Can you work these out from the model? Positions are in its coordinate system, mm. Give positions to 0.01 mm unless a question says otherwise; leave off trailing zeros. Write each loop counter-clockwise with the first axis right and the second up, starting at its lowest first coordinate (ties: lowest second). Pieces come first, ordered by that corner, then holes.
1. Suppose I cut it at D-D (y = 25.5). Please give me the cut outline in (x, z).
2. Suppose I cut it at B-B (z = 0). Please give me the cut outline in (x, y) (3 decimals), and give its area (3 significant figures).
3. Suppose I cut it at A-A (x = 0). Please give me the cut outline in (y, z), and give its area (3 significant figures).
4. Suppose I cut it at C-C (y = 4). Please give me the cut outline in (x, z).
5. I'm going to push flat-ended pins straight in: pin 1 (1 mm diameter, centred on x = 30.5, z = -13.5, fed in from -Y); pin 2 (1.5 mm diameter, centred on x = 13, z = 2, fed in from -Y); pin 3 (6 mm diameter, centred on y = 6.5, z = -28, fed in from +X). Where does each tip first touch, or does it pass through?
6. If I drill on probe 1 along Z at (x, y) = (-28.5, 18); probe 2 along Z at (x, y) = (24, 21.5); probe 3 along X at (y, z) = (14, -20), over which ranges is the centre line in solid material (lowest first)?
```python
from build123d import *

# Parameters (mm, degrees)
SKETCH_2_R          = 9
SKETCH_2_R_2        = 5.000000000000001
SKETCH_2_R_3        = 7.999999999999998
SKETCH_2_R_4        = 6.124999999999995
CUT_EXTRUDE_1_DEPTH = 107.33743200790742


with BuildPart() as part:
    # Эскиз1 → Повернуть1 (revolve)
    with BuildSketch(Plane.XY, mode=Mode.PRIVATE) as revolve_1_sk:
        with BuildLine():
            Line((0, 39.36501550915903), (0, 36.36501550915897))
            ThreePointArc((0, 36.36501550915897), (32.17757492953397, 30.613071103520923), (60.369714413268355, 14.069659601627245))
            ThreePointArc((60.369714413268355, 14.069659601627245), (65.15206854111862, 7.74515045998565), (66.84999999999997, 1.388e-14))
            Line((66.84999999999997, 1.388e-14), (69.85000000000002, 1.388e-14))
            ThreePointArc((69.85000000000002, 1.388e-14), (67.87693354038171, 9.000184617206603), (62.31964058940756, 16.349525366887885))
            ThreePointArc((62.31964058940756, 16.349525366887885), (33.216902285139106, 33.427284785509414), (0, 39.36501550915903))
        make_face()
    revolve(revolve_1_sk.sketch.rotate(Axis((0, 69.55204547466519, 0), (0, -1, 0)), 90), axis=Axis((0, 69.55204547466519, 0), (0, -1, 0)))

    # Эскиз2 → Вырез-Вытянуть1 (cut, through all)
    with BuildSketch(Plane(origin=(0, 39.36501550915903, 0), x_dir=(1, 0, 0), z_dir=(0, 1, 0))):
        with Locations(Location((0, 0, 0), (0, 0, 90))):
            Circle(SKETCH_2_R)
        with Locations(Location((-30, 0, 0), (0, 0, 137.62120169))):
            Circle(SKETCH_2_R_2)
        with Locations(Location((0, 30, 0), (0, 0, 269.99999999))):
            Circle(SKETCH_2_R_3)
        with Locations(Location((30, 0, 0), (0, 0, 136.859467324))):
            Circle(SKETCH_2_R_4)
    extrude(amount=-CUT_EXTRUDE_1_DEPTH, mode=Mode.SUBTRACT)


solid = part.part
```
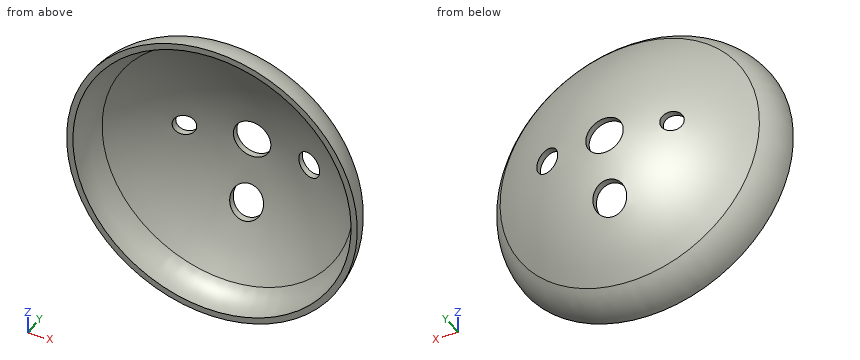
Checks:
1. outline: circle Ø99.33 at (0, 0); hole circle Ø87.18 at (0, 0)
2. outline: (-69.85, 0) - (-66.85, 0) arc R18.514 cw to (-60.37, 14.07) arc R92.88 cw to (-35, 29.518) - (-35, 32.749) arc R95.88 ccw to (-62.32, 16.35) arc R21.514 ccw to start; (-25, 32.937) arc R92.88 cw to (-9, 35.928) - (-9, 38.942) arc R95.88 ccw to (-25, 36.048) - close; (9, 35.928) arc R92.88 cw to (23.875, 33.244) - (23.875, 36.345) arc R95.88 ccw to (9, 38.942) - close; (36.125, 29.052) arc R92.88 cw to (60.37, 14.07) arc R18.514 cw to (66.85, 0) - (69.85, 0) arc R21.514 ccw to (62.32, 16.35) arc R95.88 ccw to (36.125, 32.299) - close
2. area: 380 mm2
3. outline: (0, -69.85) arc R21.51 ccw to (16.35, -62.32) arc R95.88 ccw to (31.51, -38) - (28.24, -38) arc R92.88 cw to (14.07, -60.37) arc R18.51 cw to (0, -66.85) - close; (0, 66.85) arc R18.51 cw to (14.07, 60.37) arc R92.88 cw to (35.93, 9) - (38.94, 9) arc R95.88 ccw to (16.35, 62.32) arc R21.51 ccw to (0, 69.85) - close; (33.72, -22) - (36.81, -22) arc R95.88 ccw to (38.94, -9) - (35.93, -9) arc R92.88 cw to start
3. area: 400 mm2
4. outline: circle Ø138.95 at (0, 0); hole circle Ø132.83 at (0, 0)
5. pin 1: stops at y = 29.98
5. pin 2: stops at y = 35.32
5. pin 3: stops at x = 64.44
6. probe 1: z = -53.18 to -47.56, 47.56 to 53.18
6. probe 2: z = -50.31 to -44.32, 44.32 to 50.31
6. probe 3: x = -61.5 to -57.05, 57.05 to 61.5
